from build123d import *

# Parameters (mm, degrees)
SKETCH_1_W          = 30
SKETCH_1_H          = 39.5
EXTRUDE_1_DEPTH     = 5
SKETCH_2_R          = 9
CUT_EXTRUDE_1_DEPTH = 5
SKETCH_3_W          = 17.5
SKETCH_3_H          = 30
EXTRUDE_2_DEPTH     = 3
SKETCH_6_R          = 1.5
CUT_EXTRUDE_2_DEPTH = 3


with BuildPart() as part:
    # 草图1 → 凸台-拉伸1 (new body)
    with BuildSketch(Plane(origin=(0, 0, 0), x_dir=(0, 0, -1), z_dir=(1, 0, 0))):
        with Locations((0, -8.75)):
            Rectangle(SKETCH_1_W, SKETCH_1_H)
    extrude(amount=EXTRUDE_1_DEPTH)

    # 草图2 → 切除-拉伸1 (cut)
    with BuildSketch(Plane(origin=(5, 0, 0), x_dir=(0, 0, -1), z_dir=(1, 0, 0))):
        with Locations(Location((0, -19, 0), (0, 0, 90))):
            Circle(SKETCH_2_R)
    extrude(amount=-CUT_EXTRUDE_1_DEPTH, mode=Mode.SUBTRACT)

    # 草图3 → 凸台-拉伸2 (add)
    with BuildSketch(Plane(origin=(0, 11, 0), x_dir=(1, 0, 0), z_dir=(0, 1, 0))):
        with Locations((-3.75, 0)):
            Rectangle(SKETCH_3_W, SKETCH_3_H)
    extrude(amount=EXTRUDE_2_DEPTH)

    # 草图6 → 切除-拉伸2 (cut)
    with BuildSketch(Plane(origin=(0, 14, 0), x_dir=(1, 0, 0), z_dir=(0, 1, 0))):
        with Locations(Location((-5, 10, 0), (0, 0, 270))):
            Circle(SKETCH_6_R)
        with Locations(Location((-5, -10, 0), (0, 0, 270))):
            Circle(SKETCH_6_R)
    extrude(amount=-CUT_EXTRUDE_2_DEPTH, mode=Mode.SUBTRACT)


solid = part.part
Source: CAD feature listing. Evaluate the final solid. Frame: model axes, mm. A direction names the side the tool comes from. Round coordinates to 2 decimals unless told otherwise and drop trailing zeros. Loops run counter-clockwise (first coordinate to the right, second up) from the corner with the lowest first, then second, coordinate; pieces in that order, holes last. Notation, with made-up numbers: (72.25, -7) -> (120.25, -7) arc R23 cw to (120.25, 18) -> close; hole circle Ø8 at (-11, 41). An arc over 180 degrees is marked (long way). Answer as a JSON object with one key per item and string values. Group by question number.
Q1. Section query A-A (z = 10). Output: boundary loops of the cut face in (x, y).
Q2. Section query D-D (z = 0). Output: boundary loops of the cut face in (x, y).
Q3. Section query B-B (x = -5). Output: boundary loops of the cut face in (y, z), plus the area to 3 significant figures.
Q4. Mould query, pull axis Z, two halves, no side actions, for faces 1 (the flat face through (2, -3, 15)), 2 (the flat face through (0, -4, 0)), 3 (the cylindrical face through (-4.93, 12.52, -11.5)). Classes: pulls with the +Z half, pulls with the -Z half, needs draft (parallel to the pull), parting line crosses it, or undercut.
Q5. Section query C-C (x = 0.5). Output: boundary loops of the cut face in (y, z).
Q6. Ray query, line 1 (X direction, y = 13, z = -10); line 2 (X direction, y = -3, z = 9); line 3 (Y direction, x = -0.75, z = 3). Return the intervals inside material, ascending. Write a range as from..to.
Q7. Contact query for flat-ended pins moving along their axis: P1, Ø14.5, axis at y = -19, z = 0, coming from the -X side; P2, Ø5, axis at y = -12, z = 6.5, coming from the -X side; P3, Ø5, axis at x = -7, z = 12, coming from the -Y side. Output: stop coordinate, or through.
Q8. Access query for faces 4 (the flat face through (-6, 11, 0)), 5 (the flat face through (5, -3, 0)). Directions: +Z, -Z, +X, -X, +Y, -Y. A direction counts if a zero-diameter tool reaches every point of the face in a straight line with its end or side. Return the directions, or none.
Completed:
{
 "1": {"outline": "(-12.5, 11) -> (-6.5, 11) -> (-6.5, 14) -> (-12.5, 14) -> close; (-3.5, 11) -> (0, 11) -> (0, -28.5) -> (5, -28.5) -> (5, 14) -> (-3.5, 14) -> close"},
 "2": {"outline": "(-12.5, 11) -> (0, 11) -> (0, -10) -> (5, -10) -> (5, 14) -> (-12.5, 14) -> close; (0, -28.5) -> (5, -28.5) -> (5, -28) -> (0, -28) -> close"},
 "3": {"outline": "(11, -15) -> (14, -15) -> (14, -11.5) -> (11, -11.5) -> close; (11, -8.5) -> (14, -8.5) -> (14, 8.5) -> (11, 8.5) -> close; (11, 11.5) -> (14, 11.5) -> (14, 15) -> (11, 15) -> close", "area": "72.0 mm²"},
 "4": {"face 1": "pulls with the +Z half", "face 2": "needs draft", "face 3": "undercut"},
 "5": {"outline": "(-28.5, -15) -> (14, -15) -> (14, 15) -> (-28.5, 15) -> close; hole circle Ø18 at (-19, 0)"},
 "6": {"line 1": "-12.5..-6.5, -3.5..5", "line 2": "0..5", "line 3": "11..14"},
 "7": {"P1": "through", "P2": "x = 0", "P3": "y = 11"},
 "8": {"face 4": "+Z, -Z, -X, -Y", "face 5": "+Z, -Z, +X, +Y, -Y"}
}
